The model under review builds one solid part; all positions refer to its coordinate system, in mm. A direction names the side the tool comes from. Coordinates: 2 decimals unless noted, no trailing zeros. Loops run counter-clockwise (first coordinate to the right, second up) from the corner with the lowest first, then second, coordinate; pieces in that order, holes last. Notation, with made-up numbers: (-18, 36.25) - (36, 36.25) arc R14 cw to (36, 46.25) - close; hole circle Ø5 at (62.5, -38). An arc over 180 degrees is marked (long way). Use a Markdown table: item, result. Add a question column.
1) Add section B-B, the plane y = 111.25. Give the boundary of the cut face in (x, z).
2) Clearance check with flat-ended pins moving along their axes: pin 1 (2 mm diameter, centred on x = 18, y = 115.5, fed in from +Z); pin 2 (2.5 mm diameter, centred on x = 36.28, z = 37.28, fed in from +Y); pin 3 (5.5 mm diameter, centred on x = 100.26, z = 118.32, fed in from +Y). State where each tip first meets the part, or that it passes through.
3) Add section C-C, the plane x = 52. Give the boundary of the cut face in (y, z).
4) For faces 4 (the flat face through (31.282, 111, 75)), 5 (the cylindrical face through (36.72, 114.91, 38.66)), 6 (the flat face through (75, 116.938, 41)), list the 3-axis set-ups (+Z, -Z, +X, -X, +Y, -Y) from which the entire face can be reached by the end or side of a thin tool; tool diameter is ignored.
5) Add section A-A, the plane z = 83. Give the boundary of the cut face in (x, y).
6) The part is to be moulded in two halves that separate along X. For faces 1 (the flat face through (55, 111, 24.323)), 2 (the flat face through (25, 112.938, 31)), 3 (the flat face through (110.264, 111, 74)), say which applies: pulls with the +X half, pulls with the -X half, needs draft (parallel to the pull), parting line crosses it, or undercut.
7) To check wall thickness, follow L1, parallel to X at y = 112.5, z = 81; L2, parallel to X at y = 116.75, z = 116; L3, parallel to X at y = 111, z = 31.5. State the ranges of each line that lie inside material, in increasing order. Write a range as [from, to].
```python
from build123d import *

# Parameters (mm, degrees)
SKETCH_1_R               = 3
EXTRUDE_1_DEPTH          = 4
SKETCH_2_R               = 6
SKETCH_2_R_2             = 3
SKETCH_2_R_3             = 5
SKETCH_2_R_4             = 1.45
SKETCH_2_R_5             = 3.009162644
EXTRUDE_2_DEPTH          = 4
CUT_EXTRUDE_1_DEPTH      = 167.223811286
CUT_EXTRUDE_1_DEPTH_BACK = 167.223811286
SKETCH_2_3_W             = 10
SKETCH_2_3_H             = 64.81813301
SKETCH_2_3_H_2           = 44.688768686
CHAMFER_1_SIZE           = 2


with BuildPart() as part:
    # Sketch 1 → Extrude 1 (new body)
    with BuildSketch(Plane(origin=(0, 108.938170493, 0), x_dir=(1, 0, 0), z_dir=(0, 1, 0))):
        Polygon((110.264102209, -24.322898947), (110.264102209, -124.322898947), (0.282304198, -124.322898947), (0.282304198, -24.322875098), align=None)
        with Locations(Location((10.264102209, -30.322898947, 0), (0, 0, 270))):
            Circle(SKETCH_1_R, mode=Mode.SUBTRACT)
        with Locations(Location((100.264102209, -30.322898947, 0), (0, 0, 270))):
            Circle(SKETCH_1_R, mode=Mode.SUBTRACT)
        with Locations(Location((100.264102209, -118.322898947, 0), (0, 0, 270))):
            Circle(SKETCH_1_R, mode=Mode.SUBTRACT)
        with Locations(Location((10.264102209, -118.322898947, 0), (0, 0, 270))):
            Circle(SKETCH_1_R, mode=Mode.SUBTRACT)
    extrude(amount=EXTRUDE_1_DEPTH)

    # Sketch 2 → Extrude 2 (add)
    # profile 1 of 14: a face of its own
    with BuildSketch(Plane(origin=(0, 112.938170493, 0), x_dir=(1, 0, 0), z_dir=(0, 1, 0))):
        with Locations(Location((10.264102209, -30.322898947, 0), (0, 0, 90))):
            Circle(SKETCH_2_R)
        with Locations(Location((10.264102209, -30.322898947, 0), (0, 0, 270))):
            Circle(SKETCH_2_R_2, mode=Mode.SUBTRACT)
    # profile 2 of 14: a face of its own
    with BuildSketch(Plane(origin=(0, 112.938170493, 0), x_dir=(1, 0, 0), z_dir=(0, 1, 0))):
        with Locations(Location((25.282304198, -31.322880519, 0), (0, 0, 90))):
            Circle(SKETCH_2_R_3)
        with Locations(Location((25.282304198, -31.322880519, 0), (0, 0, 270))):
            Circle(SKETCH_2_R_4, mode=Mode.SUBTRACT)
    # profile 3 of 14: a face of its own
    with BuildSketch(Plane(origin=(0, 112.938170493, 0), x_dir=(1, 0, 0), z_dir=(0, 1, 0))):
        with Locations(Location((36.282273297, -37.275706323, 0), (0, 0, 90))):
            Circle(SKETCH_2_R_3)
        with Locations(Location((36.282273297, -37.275706323, 0), (0, 0, 270))):
            Circle(SKETCH_2_R_4, mode=Mode.SUBTRACT)
    # profile 4 of 14: a face of its own
    with BuildSketch(Plane(origin=(0, 112.938170493, 0), x_dir=(1, 0, 0), z_dir=(0, 1, 0))):
        with Locations(Location((74.264102209, -39.322898947, 0), (0, 0, 90))):
            Circle(SKETCH_2_R_3)
        with Locations(Location((74.264102209, -39.322898947, 0), (0, 0, 270))):
            Circle(SKETCH_2_R_4, mode=Mode.SUBTRACT)
    # profile 5 of 14: a face of its own
    with BuildSketch(Plane(origin=(0, 112.938170493, 0), x_dir=(1, 0, 0), z_dir=(0, 1, 0))):
        with Locations(Location((100.264102209, -30.322898947, 0), (0, 0, 89.999987576))):
            Circle(SKETCH_2_R)
        with Locations(Location((100.264102209, -30.322898947, 0), (0, 0, 270))):
            Circle(SKETCH_2_R_2, mode=Mode.SUBTRACT)
    # profile 6 of 14: a face of its own
    with BuildSketch(Plane(origin=(0, 112.938170493, 0), x_dir=(1, 0, 0), z_dir=(0, 1, 0))):
        with Locations(Location((97.264102209, -49.322896128, 0), (0, 0, 90))):
            Circle(SKETCH_2_R_3)
        with Locations(Location((97.264102209, -49.322896128, 0), (0, 0, 270))):
            Circle(SKETCH_2_R_4, mode=Mode.SUBTRACT)
    # profile 7 of 14: a face of its own
    with BuildSketch(Plane(origin=(0, 112.938170493, 0), x_dir=(1, 0, 0), z_dir=(0, 1, 0))):
        with Locations(Location((98.264102209, -68.322898947, 0), (0, 0, 90))):
            Circle(SKETCH_2_R_3)
        with Locations(Location((98.264102209, -68.322898947, 0), (0, 0, 270))):
            Circle(SKETCH_2_R_4, mode=Mode.SUBTRACT)
    # profile 8 of 14: a face of its own
    with BuildSketch(Plane(origin=(0, 112.938170493, 0), x_dir=(1, 0, 0), z_dir=(0, 1, 0))):
        with Locations(Location((75.264102209, -94.322898947, 0), (0, 0, 90))):
            Circle(SKETCH_2_R_3)
        with Locations(Location((75.264102209, -94.322898947, 0), (0, 0, 270))):
            Circle(SKETCH_2_R_4, mode=Mode.SUBTRACT)
    # profile 9 of 14: a face of its own
    with BuildSketch(Plane(origin=(0, 112.938170493, 0), x_dir=(1, 0, 0), z_dir=(0, 1, 0))):
        with Locations(Location((100.264102209, -118.322898947, 0), (0, 0, 270))):
            Circle(SKETCH_2_R)
        with Locations(Location((100.264102209, -118.322898947, 0), (0, 0, 270))):
            Circle(SKETCH_2_R_2, mode=Mode.SUBTRACT)
    # profile 10 of 14: a face of its own
    with BuildSketch(Plane(origin=(0, 112.938170493, 0), x_dir=(1, 0, 0), z_dir=(0, 1, 0))):
        with Locations(Location((34.282304198, -112.822898947, 0), (0, 0, 90))):
            Circle(SKETCH_2_R_3)
        with Locations(Location((34.282304198, -112.822898947, 0), (0, 0, 270))):
            Circle(SKETCH_2_R_4, mode=Mode.SUBTRACT)
    # profile 11 of 14: a face of its own
    with BuildSketch(Plane(origin=(0, 112.938170493, 0), x_dir=(1, 0, 0), z_dir=(0, 1, 0))):
        with Locations(Location((12.782304198, -104.822898947, 0), (0, 0, 90))):
            Circle(SKETCH_2_R_3)
        with Locations(Location((12.782304198, -104.822898947, 0), (0, 0, 270))):
            Circle(SKETCH_2_R_4, mode=Mode.SUBTRACT)
    # profile 12 of 14: a face of its own
    with BuildSketch(Plane(origin=(0, 112.938170493, 0), x_dir=(1, 0, 0), z_dir=(0, 1, 0))):
        with Locations(Location((17.282304198, -69.322875098, 0), (0, 0, 90))):
            Circle(SKETCH_2_R_3)
        with Locations(Location((17.282304198, -69.322875098, 0), (0, 0, 270))):
            Circle(SKETCH_2_R_4, mode=Mode.SUBTRACT)
    # profile 13 of 14: a face of its own
    with BuildSketch(Plane(origin=(0, 112.938170493, 0), x_dir=(1, 0, 0), z_dir=(0, 1, 0))):
        with Locations(Location((25.282304198, -58.322898947, 0), (0, 0, 90))):
            Circle(SKETCH_2_R_3)
        with Locations(Location((25.282304198, -58.322898947, 0), (0, 0, 270))):
            Circle(SKETCH_2_R_4, mode=Mode.SUBTRACT)
    # profile 14 of 14: a face of its own
    with BuildSketch(Plane(origin=(0, 112.938170493, 0), x_dir=(1, 0, 0), z_dir=(0, 1, 0))):
        with Locations(Location((10.264102209, -118.322898947, 0), (0, 0, 270))):
            Circle(SKETCH_2_R)
        with Locations(Location((10.264102209, -118.322898947, 0), (0, 0, 270))):
            Circle(SKETCH_2_R_5, mode=Mode.SUBTRACT)
    extrude(amount=EXTRUDE_2_DEPTH)

    # Sketch 2_3 → Cut-Extrude 1 (cut, two sides: drawn at the far end of the back side and taken through both)
    with BuildSketch(Plane(origin=(0, 112.938170493, 0), x_dir=(1, 0, 0), z_dir=(0, 1, 0)).offset(-CUT_EXTRUDE_1_DEPTH_BACK)):
        with Locations((36.282273297, -74.684772828)):
            Rectangle(SKETCH_2_3_W, SKETCH_2_3_H)
        with Locations((74.264102209, -66.66728329)):
            Rectangle(SKETCH_2_3_W, SKETCH_2_3_H_2)
    extrude(amount=CUT_EXTRUDE_1_DEPTH + CUT_EXTRUDE_1_DEPTH_BACK, mode=Mode.SUBTRACT)

    # Chamfer 1
    chamfer_1_edges = [part.edges().sort_by_distance(p)[0] for p in [
        (10.264102209, 116.938170493, 115.313736303),
        (10.264102209, 116.938170493, 27.322898947),
        (100.264102209, 116.938170493, 27.322898947),
        (100.264102209, 116.938170493, 115.322898947),
    ]]
    chamfer(chamfer_1_edges, length=CHAMFER_1_SIZE)


solid = part.part
```
From the geometry:
| question | item | result |
|---|---|---|
| 1 | outline | (0.28, 24.32) - (110.26, 24.32) - (110.26, 124.32) - (0.28, 124.32) - close; hole circle Ø6 at (10.26, 30.32); hole circle Ø6 at (10.26, 118.32); hole (31.28, 42.28) - (41.28, 42.28) - (41.28, 107.09) - (31.28, 107.09) - close; hole (69.26, 44.32) - (79.26, 44.32) - (79.26, 89.01) - (69.26, 89.01) - close; hole circle Ø6 at (100.26, 30.32); hole circle Ø6 at (100.26, 118.32) |
| 2 | pin 1 | stops at z = 107.51 |
| 2 | pin 2 | stops at y = 112.94 |
| 2 | pin 3 | passes through |
| 3 | outline | (108.94, 24.32) - (112.94, 24.32) - (112.94, 124.32) - (108.94, 124.32) - close |
| 4 | face 4 | +Y, -Y |
| 4 | face 5 | +Y |
| 4 | face 6 | +Z, -Z, +X, -X, +Y |
| 5 | outline | (0.28, 108.94) - (31.28, 108.94) - (31.28, 112.94) - (0.28, 112.94) - close; (41.28, 108.94) - (69.26, 108.94) - (69.26, 112.94) - (41.28, 112.94) - close; (79.26, 108.94) - (110.26, 108.94) - (110.26, 112.94) - (79.26, 112.94) - close |
| 6 | face 1 | needs draft |
| 6 | face 2 | undercut |
| 6 | face 3 | pulls with the +X half |
| 7 | L1 | x = [0.28, 31.28], [41.28, 69.26], [79.26, 110.26] |
| 7 | L2 | x = [4.73, 6.04], [14.49, 15.8], [30.42, 38.14], [94.73, 96.05], [104.48, 105.8] |
| 7 | L3 | x = [0.28, 7.5], [13.02, 97.5], [103.02, 110.26] |
